from build123d import *

# Parameters (mm, degrees)
F0_R     = 41.203312
F1_DEPTH = 12.7
F2_R     = 23.225179
F3_DEPTH = 44.45
F4_R     = 35.645191
F5_DEPTH = 12.7
F6_W     = 25.4
F6_H     = 25.4
F7_DEPTH = 57.151


with BuildPart() as f1:
    # F0 (on Top) → F1 (new body)
    with BuildSketch(Plane.XY):
        Circle(F0_R)
    extrude(amount=F1_DEPTH)

    # F2 (on Top) → F3 (join)
    with BuildSketch(Plane.XY):
        Circle(F2_R)
    extrude(amount=F3_DEPTH)

    # F4 (on face) → F5 (join)
    with BuildSketch(Plane.XY.offset(44.45)):
        Circle(F4_R)
    extrude(amount=F5_DEPTH)

    # F6 (on face) → F7 (cut, through all)
    with BuildSketch(Plane.XY.offset(57.15)):
        Rectangle(F6_W, F6_H)
    extrude(amount=-F7_DEPTH, mode=Mode.SUBTRACT)


solid = f1.part
For this review, take the finished solid that the model builds, in its own axes (mm). A direction names the side the tool comes from. Round coordinates to 2 decimals unless told otherwise and drop trailing zeros. Write each loop counter-clockwise with the first axis right and the second up, starting at its lowest first coordinate (ties: lowest second). Pieces come first, ordered by that corner, then holes. Notation, with made-up numbers: (16, -29) - (67, -29) arc R33 cw to (67, 10) - close; hole circle Ø3 at (44.5, 89.5). An arc over 180 degrees is marked (long way). Use a Markdown table: item, result.
Q1. Clearance check with flat-ended pins moving along their axes: pin 1 (5 mm diameter, centred on x = 21.5, z = 44.5, fed in from -Y); pin 2 (1.5 mm diameter, centred on y = 3.5, z = 39, fed in from -X); pin 3 (1 mm diameter, centred on x = -11, y = 0.5, fed in from -Z); pin 4 (1 mm diameter, centred on y = -17, z = 9, fed in from -X). State where each tip first meets the part, or that it passes through.
Derived:
| item | result |
|---|---|
| pin 1 | stops at y = -30.16 |
| pin 2 | stops at x = -23.06 |
| pin 3 | passes through |
| pin 4 | stops at x = -37.76 |
Q2. Wall thickness on line 1 along Z through (x, y) = (25, 3); line 2 along Y through (x, z) = (0.5, 29); line 3 along Z through (x, y) = (17, 34): over which ranges is each line inside the solid? List them lowest first.
Derived:
| item | result |
|---|---|
| line 1 | z = 0 to 12.7, 44.45 to 57.15 |
| line 2 | y = -23.22 to -12.7, 12.7 to 23.22 |
| line 3 | z = 0 to 12.7 |
Q3. The part is to be moulded in two halves that separate along Z. For faces 1 (the flat face through (7, -23, 44.45)), 2 (the flat face through (15, 0, 57.15)), 3 (the flat face through (-12.7, 0, 29)), 4 (the cylindrical face through (22.15, 6.98, 28.35)), say which applies: pulls with the +Z half, pulls with the -Z half, needs draft (parallel to the pull), parting line crosses it, or undercut.
Derived:
| item | result |
|---|---|
| face 1 | undercut |
| face 2 | pulls with the +Z half |
| face 3 | needs draft |
| face 4 | undercut |
Q4. We need section D-D (y = 32). Give the boundary of the cut face in (x, z).
Derived:
| item | result |
|---|---|
| outline | (-25.96, 0) - (25.96, 0) - (25.96, 12.7) - (-25.96, 12.7) - close; (-15.7, 44.45) - (15.7, 44.45) - (15.7, 57.15) - (-15.7, 57.15) - close |
Q5. We need section B-B (z = 4). Give the boundary of the cut face in (x, y).
Derived:
| item | result |
|---|---|
| outline | circle Ø82.41 at (0, 0); hole (-12.7, -12.7) - (12.7, -12.7) - (12.7, 12.7) - (-12.7, 12.7) - close |
Q6. We need section A-A (y = 0). Give the boundary of the cut face in (x, z), plus the area to 3 significant figures.
Derived:
| item | result |
|---|---|
| outline | (-41.2, 0) - (-12.7, 0) - (-12.7, 57.15) - (-35.65, 57.15) - (-35.65, 44.45) - (-23.23, 44.45) - (-23.23, 12.7) - (-41.2, 12.7) - close; (12.7, 0) - (41.2, 0) - (41.2, 12.7) - (23.23, 12.7) - (23.23, 44.45) - (35.65, 44.45) - (35.65, 57.15) - (12.7, 57.15) - close |
| area | 1,980 mm2 |
Q7. Machinability: for faces 5 (the flat face through (12.7, 0, 29)), 6 (the flat face through (18, -18, 12.7)), 7 (the cylindrical face through (-4.64, 35.34, 50.71)), which of the approach directions +Z, -Z, +X, -X, +Y, -Y give a long, thin tool a straight path to every point of the face, cutting with its end or side? Answer none if there is none.
Derived:
| item | result |
|---|---|
| face 5 | +Z, -Z |
| face 6 | none |
| face 7 | +Z |
